from build123d import *

# Parameters (mm, degrees)
SKETCH1_R           = 50
BOSS_EXTRUDE1_DEPTH = 25
SKETCH2_R           = 10
BOSS_EXTRUDE2_DEPTH = 20
BOSS_EXTRUDE3_START = 20
SKETCH3_R           = 10
BOSS_EXTRUDE3_DEPTH = 20


with BuildPart() as part:
    # Sketch1 → Boss-Extrude1 (new, symmetric)
    with BuildSketch(Plane.XY):
        Circle(SKETCH1_R)
    extrude(amount=BOSS_EXTRUDE1_DEPTH, both=True)

    # Sketch2 → Boss-Extrude2 (add)
    with BuildSketch(Plane(origin=(0, 0, -25), x_dir=(-1, 0, 0), z_dir=(0, 0, -1))):
        Circle(SKETCH2_R)
    extrude(amount=BOSS_EXTRUDE2_DEPTH)

    # Sketch3 → Boss-Extrude3 (add)
    with BuildSketch(Plane.XY.offset(25).offset(BOSS_EXTRUDE3_START)):
        with Locations(Location((0, 0, 0), (0, 0, 180))):
            Circle(SKETCH3_R)
    extrude(amount=-BOSS_EXTRUDE3_DEPTH)


solid = part.part
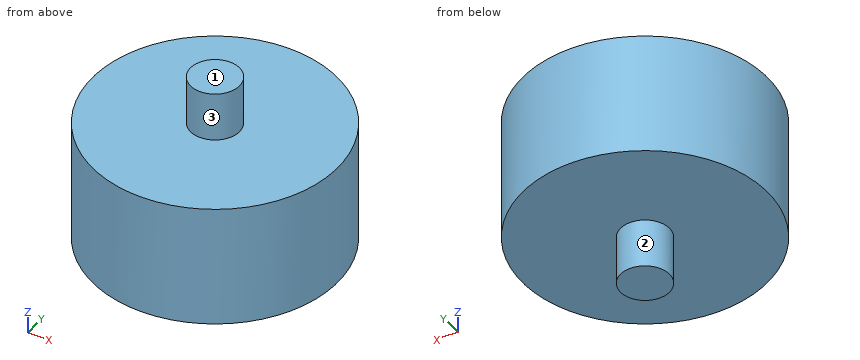
Could you check a few things on this model? Use its own coordinates, in mm. Face numbers are marked on the shaded views. A direction names the side the tool comes from. Round coordinates to 2 decimals unless told otherwise and drop trailing zeros. Write each loop counter-clockwise with the first axis right and the second up, starting at its lowest first coordinate (ties: lowest second). Pieces come first, ordered by that corner, then holes. Notation, with made-up numbers: (-17, 1.5) - (-7, 1.5) arc R14 ccw to (-7, 12.5) - close; hole circle Ø7 at (56.5, 81.5). An arc over 180 degrees is marked (long way). Use a Markdown table: item, result.
Q1. Please list where these lines run through material, in increasing order: L1, parallel to Z at x = -15, y = 15.5; L2, parallel to X at y = -29, z = 10.5; L3, parallel to X at y = -44, z = 4.5.
Output values:
| item | result |
|---|---|
| L1 | -25 to 25 |
| L2 | -40.73 to 40.73 |
| L3 | -23.75 to 23.75 |
Q2. I want a section at C-C (z = -31). List the corners of the cut face in (x, y) for me, plus the area to 3 significant figures.
Output values:
| item | result |
|---|---|
| outline | circle Ø20 at (0, 0) |
| area | 314 mm2 |
Q3. I want a section at A-A (x = 0). List the corners of the cut face in (y, z) for me.
Output values:
| item | result |
|---|---|
| outline | (-50, -25) - (-10, -25) - (-10, -45) - (10, -45) - (10, -25) - (50, -25) - (50, 25) - (10, 25) - (10, 45) - (-10, 45) - (-10, 25) - (-50, 25) - close |
Q4. For pin 1 (2 mm diameter, centred on x = 17, z = -11, fed in from +Y); pin 2 (4 mm diameter, centred on y = -27, z = -9.5, fed in from -X); pin 3 (10 mm diameter, centred on x = 3.5, z = 24.5, fed in from +Y), each with a flat end and sliding along its axis, tell me the tip position at first contact or that it passes through.
Output values:
| item | result |
|---|---|
| pin 1 | y = 47.37 |
| pin 2 | x = -43.3 |
| pin 3 | y = 50 |
Q5. For the marked faces 1, 2 and 3, which set-ups out of +Z, -Z, +X, -X, +Y, -Y let a thin tool reach every point of the face, with its end or its side?
Output values:
| item | result |
|---|---|
| face 1 | +Z, +X, -X, +Y, -Y |
| face 2 | -Z |
| face 3 | +Z |
Q6. I want a section at D-D (x = -30). List the corners of the cut face in (y, z) for me, plus the area to 3 significant figures.
Output values:
| item | result |
|---|---|
| outline | (-40, -25) - (40, -25) - (40, 25) - (-40, 25) - close |
| area | 4,000 mm2 |
